Verification items for the finished model (mm, model axes). A direction names the side the tool comes from. Give positions to 0.01 mm unless a question says otherwise; leave off trailing zeros. Order: outer loops, then holes, each group sorted by start corner. A loop starts at its lowest first (then second) coordinate and runs counter-clockwise, first axis right, second up. Notation, with made-up numbers: M 61.5,-32.5 L 73.5,-32.5 A22 cw 73.5,-8.5 Z; hole C 28,12.5 d7. An arc over 180 degrees is marked long. Answer as a JSON object with one key per item and string values.
Autodesk Inventor part; units mm, degrees
ref_plane "YZ Plane" through (0, 0, 0) normal (1, 0, 0) x (0, 1, 0)
ref_plane "XZ Plane" through (0, 0, 0) normal (0, 1, 0) x (-1, 0, 0)
ref_plane "XY Plane" through (0, 0, 0) normal (0, 0, 1) x (1, 0, 0)
sketch "Эскиз1" plane through (0, 0, 0) normal (0, 1, 0) x (-1, 0, 0)
  line L0 (0, 0) -> (6.7, 0)
  line L1 (6.7, 0) -> (6.7, 2.7)
  line L2 (6.7, 2.7) -> (0, 2.7)
  line L3 (0, 2.7) -> (0, 0)
  dimension "d0" = 6.7
  dimension "d1" = 2.7
extrude "Выдавливание1" add sketch "Эскиз1" against normal blind 1.4
sketch "Эскиз2" plane through (0, 0, 0) normal (0, 1, 0) x (1, 0, 0)
  line L0 (0, 0) -> (-6.7, 0)
  circle A0 centre (-4.85, -1.35) radius 0.35
  circle A1 centre (-1.85, -1.35) radius 0.35
  point P0 (0, -2.7)
  dimension "d4" = 0.7
  dimension "d6" = 1.35
  dimension "d7" = 2.7
  dimension "d9" = 1.35
  dimension "d10" = 3
  dimension "d11" = 1.85
  dimension "d12" = 6.7
extrude "Выдавливание2" add sketch "Эскиз2" along normal blind 0.5
sketch "Эскиз3" plane through (-6.7, 0, 2.7) normal (0, 0, 1) x (1, 0, 0)
  line L0 (0, 0) -> (6.7, 0)
  line L1 (1.9, -0.05) -> (3.2, -0.05)
  line L2 (3.2, -0.05) -> (3.2, -1.35)
  line L3 (3.2, -1.35) -> (1.9, -1.35)
  line L4 (1.9, -1.35) -> (1.9, -0.05)
  line L5 (1.85, -0.05) -> (4.85, -0.05)
  line L6 (4.85, -0.05) -> (4.85, -1.35)
  line L7 (4.85, -1.35) -> (1.85, -1.35)
  line L8 (1.85, -1.35) -> (1.85, -0.05)
  line L9 (3.5, -0.05) -> (4.8, -0.05)
  line L10 (4.8, -0.05) -> (4.8, -1.35)
  line L11 (4.8, -1.35) -> (3.5, -1.35)
  line L12 (3.5, -1.35) -> (3.5, -0.05)
  point P0 (0, -1.4)
  point P1 (6.7, -1.4)
  dimension "d15" = 1.3
  dimension "d16" = 1.3
  dimension "d18" = 0.05
  dimension "d20" = 3
  dimension "d21" = 1.3
  dimension "d22" = 1.85
  dimension "d23" = 6.7
  dimension "d24" = 0.05
  dimension "d25" = 0.05
  dimension "d51" = 1.3
  dimension "d52" = 1.3
  dimension "d53" = 0.05
extrude "Выдавливание3" add sketch "Эскиз3" along normal blind 1.5 contours L1 L2 L3 L4
sketch "Эскиз4" plane through (0, 0, 0) normal (0, 1, 0) x (1, 0, 0)
  line L0 (0, 0) -> (0.55, 0)
  line L1 (0.55, 0) -> (0.55, -0.4)
  line L2 (0.55, -0.4) -> (0, -0.4)
  line L3 (0, -0.4) -> (0, 0)
  line L4 (0, -2.7) -> (0.55, -2.7)
  line L5 (0.55, -2.7) -> (0.55, -2.3)
  line L6 (0.55, -2.3) -> (0, -2.3)
  line L7 (0, -2.3) -> (0, -2.7)
  line L8 (-6.7, -2.7) -> (-7.25, -2.7)
  line L9 (-7.25, -2.7) -> (-7.25, -2.3)
  line L10 (-7.25, -2.3) -> (-6.7, -2.3)
  line L11 (-6.7, -2.3) -> (-6.7, -2.7)
  line L12 (-6.7, 0) -> (-7.25, 0)
  line L13 (-7.25, 0) -> (-7.25, -0.4)
  line L14 (-7.25, -0.4) -> (-6.7, -0.4)
  line L15 (-6.7, -0.4) -> (-6.7, 0)
  dimension "d28" = 0.55
  dimension "d29" = 0.4
  dimension "d30" = 0.4
  dimension "d31" = 0.55
  dimension "d32" = 0.4
  dimension "d33" = 0.4
extrude "Выдавливание4" add sketch "Эскиз4" against normal blind 0.15
fillet "Сопряжение1" radius 0.1 2 edges at (-5.2, 0.5, 1.35) (-2.2, 0.5, 1.35)
fillet "Сопряжение2" radius 0.1 8 edges at (-4.8, -0.05, 3.45) (-3.5, -0.05, 3.45) (-4.15, -0.05, 4.2) (-4.15, -1.35, 4.2) (-3.5, -0.7, 4.2) (-3.5, -1.35, 3.45) (-4.8, -1.35, 3.45) (-4.8, -0.7, 4.2)
fillet "Сопряжение2" radius 0.1 2 edges at (-4.15, -0.05, 4.2) (-4.15, -1.35, 4.2)
sketch "Эскиз6" plane through (-6.7, -1.4, 2.7) normal (0, 0, 1) x (1, 0, 0)
  line L0 (3.2, 1.25) -> (3.2, 0.15)
  arc A0 (3.1, 0.05) -> (3.2, 0.15) centre (3.1, 0.15) ccw
  arc A1 (1.9, 0.15) -> (2, 0.05) centre (2, 0.15) ccw
  line L1 (1.9, 0.15) -> (1.9, 1.25)
  arc A2 (2, 1.35) -> (1.9, 1.25) centre (2, 1.25) ccw
  arc A3 (3.2, 1.25) -> (3.1, 1.35) centre (3.1, 1.25) ccw
  line L2 (0, 0) -> (6.7, 0)
  line L3 (1.85, 1.35) -> (4.85, 1.35)
  line L4 (4.85, 1.35) -> (4.85, 0.05)
  line L5 (1.85, 0.05) -> (1.85, 1.35)
  line L6 (4.85, 0.05) -> (1.85, 0.05)
extrude "Выдавливание5" cut sketch "Эскиз6" against normal blind 0.1 contours A3 L3 L4 L6 A0 L0 | A2 L1 A1 L6 L5 L3
sketch "Эскиз7" plane through (0, 0, 0) normal (0, 1, 0) x (1, 0, 0)
  circle A0 centre (-4.85, -1.35) radius 0.35
  circle A1 centre (-1.85, -1.35) radius 0.35
  line L0 (0.55, 0) -> (-7.25, 0)
  line L1 (-7.25, 0) -> (-7.25, -0.4)
  line L2 (-7.25, -0.4) -> (-6.7, -0.4)
  line L3 (-6.7, -0.4) -> (-6.7, -2.3)
  line L4 (-6.7, -2.3) -> (-7.25, -2.3)
  line L5 (-7.25, -2.3) -> (-7.25, -2.7)
  line L6 (-7.25, -2.7) -> (0.55, -2.7)
  line L7 (0.55, -2.7) -> (0.55, -2.3)
  line L8 (0.55, -2.3) -> (0, -2.3)
  line L9 (0, -2.3) -> (0, -0.4)
  line L10 (0, -0.4) -> (0.55, -0.4)
  line L11 (0.55, -0.4) -> (0.55, 0)
  point P0 (0, 0)
  dimension "d49" = 1.35
  dimension "d50" = 3
sketch "Эскиз8" plane through (-6.7, -1.4, 2.7) normal (0, 0, 1) x (1, 0, 0)
  line L0 (1.85, 1.35) -> (2, 1.35)
  line L1 (2, 1.35) -> (3.1, 1.35)
  line L2 (3.1, 1.35) -> (2, 1.35)
  line L3 (3.6, 1.35) -> (4.7, 1.35)
  line L4 (1.85, 1.35) -> (4.85, 1.35)
  line L5 (4.85, 1.35) -> (4.85, 0.05)
  line L6 (4.85, 0.05) -> (3.1, 0.05)
  line L7 (4.7, 0.05) -> (3.6, 0.05)
  line L8 (4.85, 0.05) -> (3.1, 0.05)
  line L9 (3.1, 0.05) -> (2, 0.05)
  line L10 (2, 0.05) -> (1.85, 0.05)
  line L11 (1.85, 0.05) -> (1.85, 1.35)
equation "\"d6\" = 0.5 * d7"
equation "\"d9\" = d6"
equation "\"d11\" = -0.5 * d10 + 0.5 * d12"
equation "\"d22\" = -0.5 * d20 + 0.5 * d23"
properties part number "msk12c02"
Q1. Release check for a two-part mould opening along X. For faces 4 (the face through (-3, -1, 2.6)), 5 (the face through (-4, -1, 4.2)) record: +X half, -X half, draft (parallel to the pull), parting line (faces both ways), or undercut.
Resolved:
{"face 4": "undercut", "face 5": "draft"}
Q2. Section check D-D on z = 1.35. Record the cut outline in (x, y), then the cut area to 3 significant figures.
Resolved:
{"outline": "M -6.7,-1.4 L 0,-1.4 L 0,0 L -1.5,0 L -1.5,0.4 A0.1 ccw -1.6,0.5 L -2.1,0.5 A0.1 ccw -2.2,0.4 L -2.2,0 L -4.5,0 L -4.5,0.4 A0.1 ccw -4.6,0.5 L -5.1,0.5 A0.1 ccw -5.2,0.4 L -5.2,0 L -6.7,0 Z", "area": "10.1 mm²"}
Q3. Section check A-A on z = 3.1. Record the cut outline in (x, y).
Resolved:
{"outline": "M -4.8,-1.25 A0.1 ccw -4.7,-1.35 L -3.6,-1.35 A0.1 ccw -3.5,-1.25 L -3.5,-0.15 A0.1 ccw -3.6,-0.05 L -4.7,-0.05 A0.1 ccw -4.8,-0.15 Z"}
Q4. Section check B-B on y = -0.7. Record the cut outline in (x, z), then the cut area to 3 significant figures.
Resolved:
{"outline": "M -6.7,0 L 0,0 L 0,2.7 L -1.85,2.7 L -1.85,2.6 L -3.5,2.6 L -3.5,4.1 A0.1 ccw -3.6,4.2 L -4.7,4.2 A0.1 ccw -4.8,4.1 L -4.8,2.6 L -4.85,2.6 L -4.85,2.7 L -6.7,2.7 Z", "area": "19.9 mm²"}
Q5. Section check C-C on x = -3.25. Record the cut outline in (y, z), then the cut area to 3 significant figures.
Resolved:
{"outline": "M -1.4,0 L 0,0 L 0,2.7 L -0.05,2.7 L -0.05,2.6 L -1.35,2.6 L -1.35,2.7 L -1.4,2.7 Z", "area": "3.65 mm²"}
Q6. Gauge pin test, flat ends, axial feed: pin 1 Ø1.2 at (x, z) = (-4, 3.5) entering from -Y; pin 2 Ø1.2 at (x, z) = (-4.5, 3.5) entering from +Y; pin 3 Ø0.7 at (y, z) = (-0.5, 1.5) entering from +X. Record the tip position at first contact, or that the pin passes through.
Resolved:
{"pin 1": "stops at y = -1.35", "pin 2": "stops at y = -0.05", "pin 3": "stops at x = 0"}
Q7. Tool access check on faces 1 (the face through (-3, -1, 0)), 2 (the face through (-4, -1.35, 3)), 3 (the face through (-4, -0.05, 3)). Record the directions out of +Z, -Z, +X, -X, +Y, -Y that give a thin tool (end or side, any length) a straight path to the whole face; none if there is none.
Resolved:
{"face 1": "-Z, +X, -X, +Y, -Y", "face 2": "+Z, +X, -X, -Y", "face 3": "+Z, +X, -X, +Y"}
Q8. Material ranges on L1, parallel to Z at x = -2.5, y = -0.1; L2, parallel to X at y = -0.9, z = 3.1; L3, parallel to Y at x = -1, z = 0.4, recorded low to high.
Resolved:
{"L1": "z = 0 to 2.6", "L2": "x = -4.8 to -3.5", "L3": "y = -1.4 to 0"}
